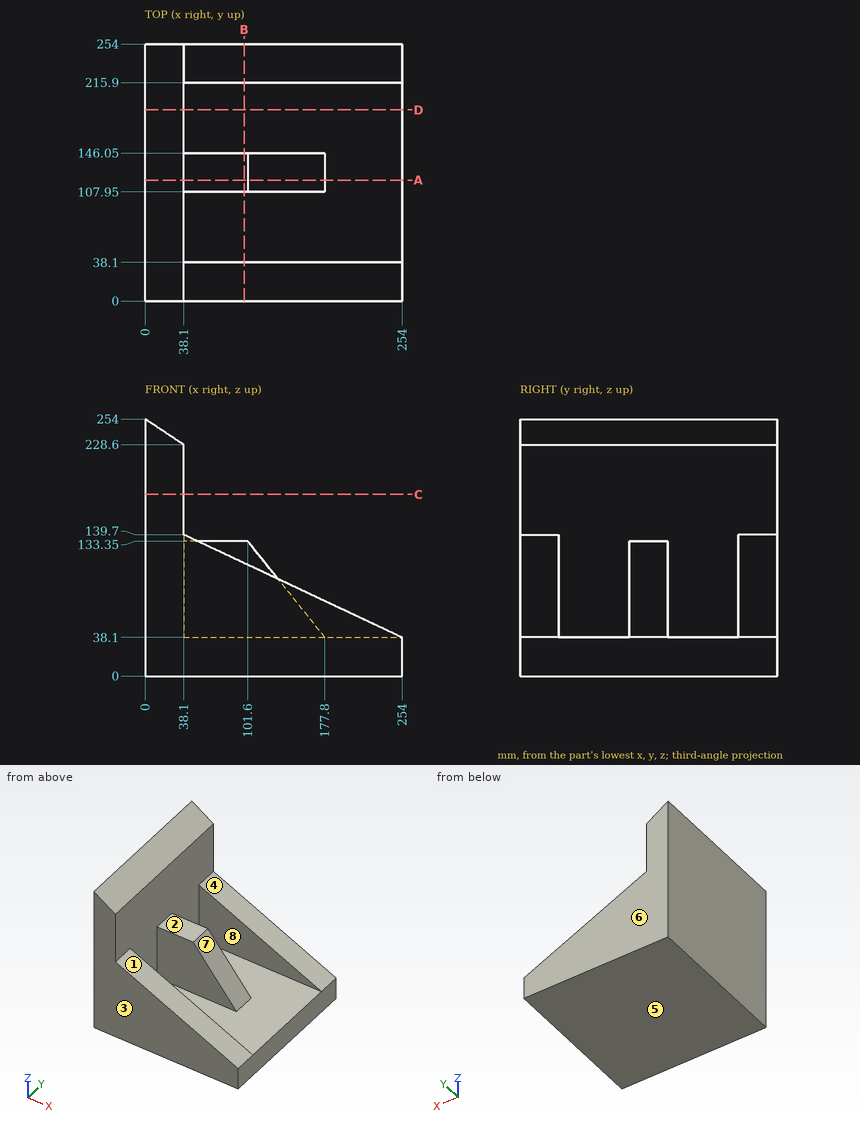
Can you work these out from the drawing? Everything is in mm from the part's minimum corner. A direction names the side the tool comes from. Round coordinates to 2 decimals unless told otherwise and drop trailing zeros. Order: outer loops, then holes, each group sorted by start corner. A loop starts at its lowest first (then second) coordinate and runs counter-clockwise, first axis right, second up. Notation, with made-up numbers: (79, -9.75) -> (127, -9.75) arc R21 ccw to (127, 12.25) -> close; hole circle Ø3 at (13, 43). An arc over 180 degrees is marked (long way). Return JSON: item names as keys, results as strings. Group by question number.
1. If we section it at D-D, the plane y = 189: Write out the boundary of the cut face in (x, z), then the cut area to 3 significant figures.
2. If we section it at C-C, the plane z = 179.5: Write out the boundary of the cut face in (x, y).
3. We'd pull the mould along Y, two halves only. Please class the marked faces 5, 6, 7 and 8: released by +Y, released by -Y, zero draft, split by the parting line, or undercut.
4. If we section it at B-B, the plane x = 98: Write out the boundary of the cut face in (y, z), then the cut area to 3 significant figures.
5. Which directions (+Z, -Z, +X, -X, +Y, -Y) give clear straight access to the entire face, cutting with the end or side of a thin tool? Please do the marked faces 1, 2, 3 and 4.
6. Will these pins go through, and if not, where does the flat tip stop? pin 1 (1.5 mm diameter, centred on y = 43, z = 53, fed in from +X); pin 2 (8 mm diameter, centred on x = 53.5, y = 155.5, fed in from +Z); pin 3 (8 mm diameter, centred on x = 37, z = 82, fed in from -Y).
7. If we section it at A-A, the plane y = 119.5: Write out the boundary of the cut face in (x, z), then the cut area to 3 significant figures.
8. I need wall thicknesses on line 1 (Y direction, x = 52, z = 82); line 2 (Z direction, x = 126, y = 62). Which ranges of each line are inside material? Lowest first, please. Write a range as [from, to].
Output values:
{
 "1": {"outline": "(0, 0) -> (254, 0) -> (254, 38.1) -> (38.1, 38.1) -> (38.1, 228.6) -> (0, 254) -> close", "area": "17,400 mm²"},
 "2": {"outline": "(0, 0) -> (38.1, 0) -> (38.1, 254) -> (0, 254) -> close"},
 "3": {"face 5": "zero draft", "face 6": "released by +Y", "face 7": "undercut", "face 8": "undercut"},
 "4": {"outline": "(0, 0) -> (254, 0) -> (254, 111.51) -> (215.9, 111.51) -> (215.9, 38.1) -> (146.05, 38.1) -> (146.05, 133.35) -> (107.95, 133.35) -> (107.95, 38.1) -> (38.1, 38.1) -> (38.1, 111.51) -> (0, 111.51) -> close", "area": "18,900 mm²"},
 "5": {"face 1": "+Z, +X, -Y", "face 2": "+Z, +X", "face 3": "+Z, -Z, +X, -X, -Y", "face 4": "+Z, +X, +Y"},
 "6": {"pin 1": "x = 38.1", "pin 2": "z = 38.1", "pin 3": "y = 0"},
 "7": {"outline": "(0, 0) -> (254, 0) -> (254, 38.1) -> (177.8, 38.1) -> (101.6, 133.35) -> (38.1, 133.35) -> (38.1, 228.6) -> (0, 254) -> close", "area": "27,100 mm²"},
 "8": {"line 1": "[0, 38.1], [107.95, 146.05], [215.9, 254]", "line 2": "[0, 38.1]"}
}
